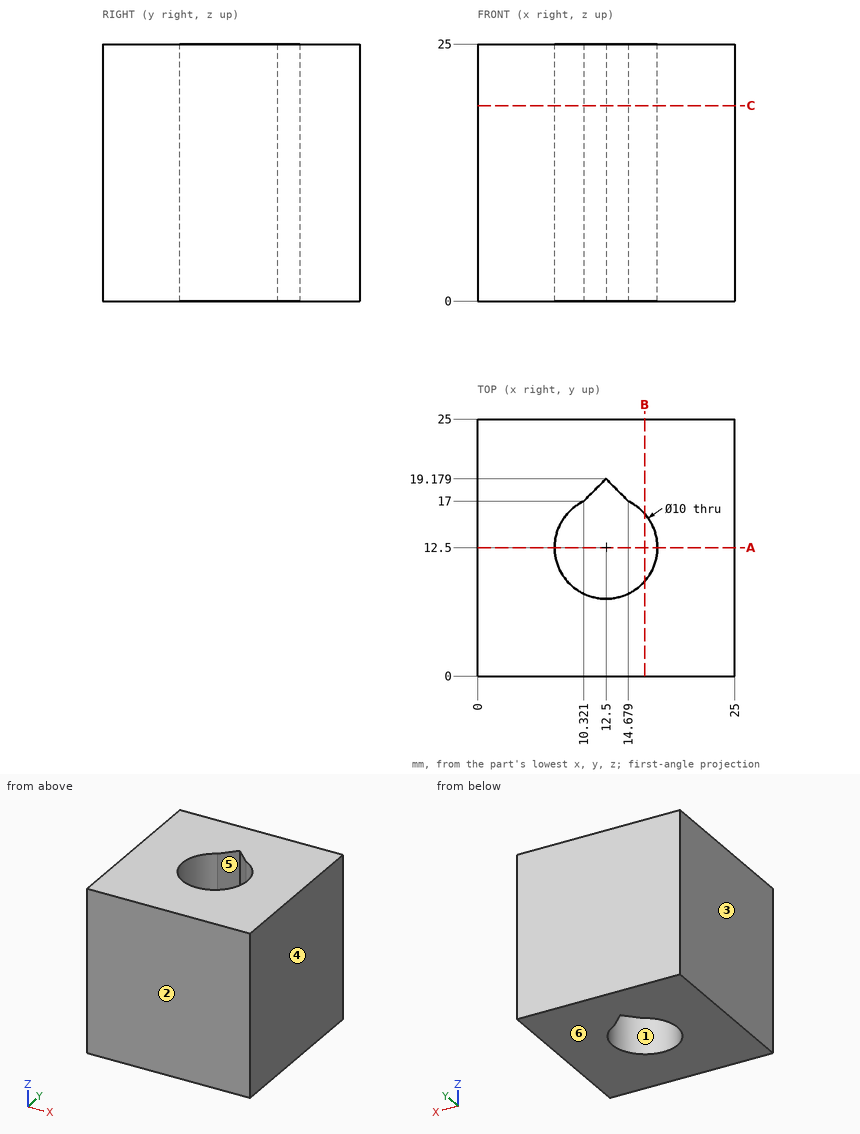
Input: dimensioned drawing with shaded views. Units: mm. Origin: part minimum x, y, z. A direction names the side the tool comes from. Coordinates: 2 decimals unless noted, no trailing zeros. Loops run counter-clockwise (first coordinate to the right, second up) from the corner with the lowest first, then second, coordinate; pieces in that order, holes last. Notation, with made-up numbers: (47, 88.25) -> (102, 88.25) arc R9 cw to (102, 93.25) -> close; hole circle Ø9 at (14.25, -18.5). An arc over 180 degrees is marked (long way). One line per item, written item: value. Start each with the question number.
Q1. Set-up query: the marked faces 5 and 6. Return all of +Z, -Z, +X, -X, +Y, -Y with unobstructed straight access to the full face (end or side cutting, diameter ignored); none if empty.
Q2. Mould query, pull axis X, two halves, no side actions, for the marked faces 1, 2, 3 and 4. Classes: pulls with the +X half, pulls with the -X half, needs draft (parallel to the pull), parting line crosses it, or undercut.
Q3. Section query C-C, the plane z = 19. Return the cut outline in (x, y).
Q4. Section query B-B, the plane x = 16.25. Return the cut outline in (y, z).
Q5. Contact query for a flat-ended pin moving along its axis: P1, Ø13, axis at x = 12.5, y = 12.5, coming from the -Z side. Output: stop coordinate, or through.
Q6. Line query: line 1 along X through (y, z) = (12.25, 3.25); line 2 along Y through (x, z) = (17, 5.5) (1 decimal); line 3 along X through (y, z) = (9, 19.5). Output: solid intervals per line, ascending.
Q7. Section query A-A, the plane y = 12.5. Return the cut outline in (x, z).
Results:
1. face 5: +Z, -Z
1. face 6: -Z, +X, -X, +Y, -Y
2. face 1: undercut
2. face 2: needs draft
2. face 3: pulls with the -X half
2. face 4: pulls with the +X half
3. outline: (0, 0) -> (25, 0) -> (25, 25) -> (0, 25) -> close; hole (10.32, 17) arc R5 ccw (long way) to (14.68, 17) -> (12.5, 19.18) -> close
4. outline: (0, 0) -> (9.19, 0) -> (9.19, 25) -> (0, 25) -> close; (15.81, 0) -> (25, 0) -> (25, 25) -> (15.81, 25) -> close
5. P1: z = 0
6. line 1: 0 to 7.51, 17.49 to 25
6. line 2: 0 to 10.3, 14.7 to 25
6. line 3: 0 to 8.93, 16.07 to 25
7. outline: (0, 0) -> (7.5, 0) -> (7.5, 25) -> (0, 25) -> close; (17.5, 0) -> (25, 0) -> (25, 25) -> (17.5, 25) -> close
